Can you work these out from the drawing? Everything is in mm from the part's minimum corner. Coordinates: 2 decimals unless noted, no trailing zeros. Loops run counter-clockwise (first coordinate to the right, second up) from the corner with the lowest first, then second, coordinate; pieces in that order, holes last. Notation, with made-up numbers: M -18,-26.5 L 25,-26.5 A34 cw 25,8.5 Z; hole C 78.5,-27.5 d3. An arc over 180 degrees is marked long. Use CSV: the item, a comma, the result in double quotes. Start each with the question number.
Q1. If we section it at B-B (x = 14): Please give me the cut outline in (y, z).
Q2. For pin 1 Ø1 at (x, y) = (23.5, 5) entering from -Z; pin 2 Ø2 at (x, z) = (7.5, 2) entering from -Y; pin 3 Ø3 at (x, y) = (11, 3.5) entering from -Z, each with a flat end and sliding along its axis, tell me the tip position at first contact or that it passes through.
Q3. Please list where these lines run through material, in increasing order: probe 1 along Y at (x, z) = (17, 1) (1 decimal); probe 2 along Y at (x, z) = (14, 3.5) (1 decimal); probe 3 along X at (y, z) = (7.5, 2.5). Write a range as [from, to].
Q4. If we section it at A-A (y = 6): Please give me the cut outline in (x, z).
Q5. If we mould it in two halves opening along X, with no side actions, what happens to the marked faces 1, 2 and 3? For each: +X half, -X half, draft (parallel to the pull), parting line (faces both ways), or undercut.
Q6. If we section it at D-D (y = 7.5): Please give me the cut outline in (x, z).
Q7. If we section it at C-C (z = 2): Please give me the cut outline in (x, y).
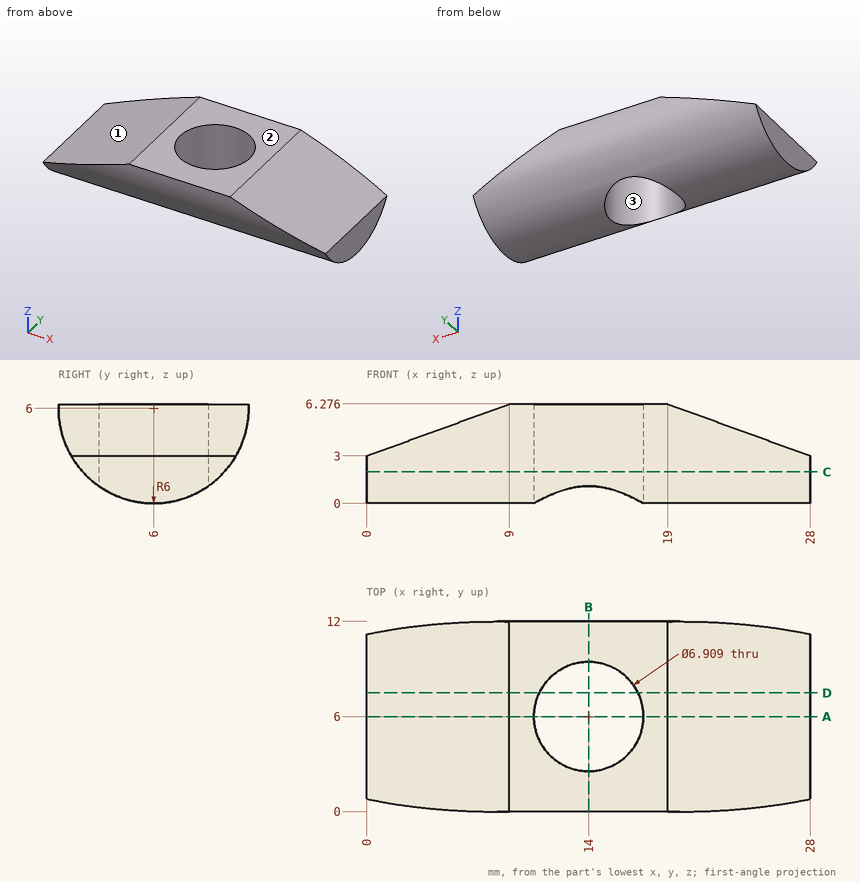
Results below:
1,outline,"M 0.01,6.28 A6 ccw 2.55,1.09 L 2.55,6.28 Z; M 9.45,1.09 A6 ccw 11.99,6.28 L 9.45,6.28 Z"
2,pin 1,"z = 0.02"
2,pin 2,"y = 0.8"
2,pin 3,"z = 0.09"
3,probe 1,"[2.7, 4.3], [7.7, 9.3]"
3,probe 2,"[0.5, 2.5], [9.5, 11.5]"
3,probe 3,"[0, 10.89], [17.11, 28]"
4,outline,"M 0,0 L 10.55,0 L 10.55,6.28 L 9,6.28 L 0,3 Z; M 17.45,0 L 28,0 L 28,3 L 19,6.28 L 17.45,6.28 Z"
5,face 1,"-X half"
5,face 2,"draft"
5,face 3,"undercut"
6,outline,"M 0,0.19 L 10.89,0.19 L 10.89,6.28 L 9,6.28 L 0,3 Z; M 17.11,0.19 L 28,0.19 L 28,3 L 19,6.28 L 17.11,6.28 Z"
7,outline,"M 0,1.53 L 28,1.53 L 28,10.47 L 0,10.47 Z; hole C 14,6 d6.91"
